The drawing under review shows one solid part. Ordinate dimensions are in mm from its lowest x, y, z. Coordinates: 2 decimals unless noted, no trailing zeros. Loops run counter-clockwise (first coordinate to the right, second up) from the corner with the lowest first, then second, coordinate; pieces in that order, holes last. Notation, with made-up numbers: (50.5, -12.75) -> (64.5, -12.75) arc R27 ccw to (64.5, 13.25) -> close; hole circle Ø7 at (-26, 6.5). An arc over 180 degrees is marked (long way). Use a Markdown table: item, result.
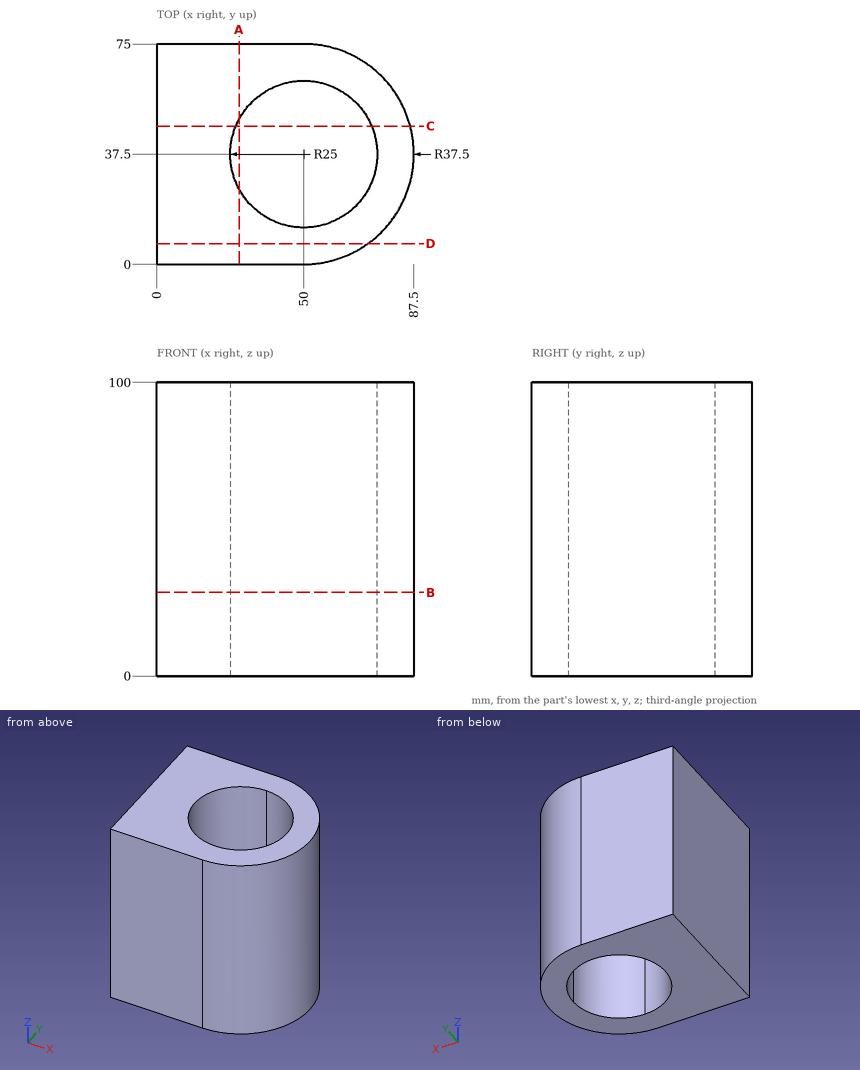
(1) Take a section at D-D on y = 7. Write out the cut boundary in (x, z), plus the area to 3 significant figures.
Found:
| item | result |
|---|---|
| outline | (0, 0) -> (71.82, 0) -> (71.82, 100) -> (0, 100) -> close |
| area | 7,180 mm^2 |
(2) For pin 1 Ø5 at (y, z) = (17.5, 20) entering from +X; pin 2 Ø1 at (y, z) = (45, 25) entering from +X; pin 3 Ø12 at (y, z) = (26, 11.5) entering from +X, all flat-tipped, find the tip position at first contact; note any pin that passes through.
Found:
| item | result |
|---|---|
| pin 1 | stops at x = 83.17 |
| pin 2 | stops at x = 86.84 |
| pin 3 | stops at x = 87.09 |
(3) For line 1 along Y through (x, z) = (51, 65); line 2 along X through (y, z) = (38.5, 65.5); line 3 along Y through (x, z) = (61, 95), list the stretches that pass through material, from the lowest coordinate up.
Found:
| item | result |
|---|---|
| line 1 | y = 0.01 to 12.52, 62.48 to 74.99 |
| line 2 | x = 0 to 25.02, 74.98 to 87.49 |
| line 3 | y = 1.65 to 15.05, 59.95 to 73.35 |
(4) Take a section at C-C on y = 47. Write out the cut boundary in (x, z), plus the area to 3 significant figures.
Found:
| item | result |
|---|---|
| outline | (0, 0) -> (26.88, 0) -> (26.88, 100) -> (0, 100) -> close; (73.12, 0) -> (86.28, 0) -> (86.28, 100) -> (73.12, 100) -> close |
| area | 4,000 mm^2 |
(5) Take a section at B-B on z = 28.5. Write out the cut boundary in (x, y).
Found:
| item | result |
|---|---|
| outline | (0, 0) -> (50, 0) arc R37.5 ccw to (50, 75) -> (0, 75) -> close; hole (50, 12.5) arc R25 ccw to (75, 37.5) arc R25 ccw to (50, 62.5) arc R25 ccw to start |
(6) Take a section at A-A on x = 28. Write out the cut boundary in (y, z).
Found:
| item | result |
|---|---|
| outline | (0, 0) -> (25.63, 0) -> (25.63, 100) -> (0, 100) -> close; (49.37, 0) -> (75, 0) -> (75, 100) -> (49.37, 100) -> close |
